The drawing under review shows one solid part. Ordinate dimensions are in mm from its lowest x, y, z. A direction names the side the tool comes from. Coordinates: 2 decimals unless noted, no trailing zeros. Write each loop counter-clockwise with the first axis right and the second up, starting at its lowest first coordinate (ties: lowest second). Pieces come first, ordered by that corner, then holes. Notation, with made-up numbers: (63.25, 43.5) -> (74.25, 43.5) arc R20 ccw to (74.25, 64.5) -> close; hole circle Ø9 at (-9.5, 22.25). An arc over 180 degrees is marked (long way). One line per question, with ' | ' between items. Start each with the question number.
Q1. Add section A-A on y = 95.5. State the section outline as (x, z) points (3 decimals).
Q2. Wall thickness on probe 1 along Y at (x, z) = (10.5, 54.5) (3 decimals); probe 2 along Z at (x, y) = (18, 133.5); probe 3 along Z at (x, y) = (13.25, 130.5): over which ranges is each line inside the solid? List them lowest first.
Q3. Draft analysis for pull direction Y (two halves, no side actions). For the marked faces 3, 4 and 5, state which applies: pulls with the +Y half, pulls with the -Y half, needs draft (parallel to the pull), parting line crosses it, or undercut.
Q4. Add section B-B on x = 9.25. State the section outline as (y, z) points (3 decimals), and give its area (3 significant figures).
Q5. For the marked faces 1 and 2, list the 3-axis set-ups (+Z, -Z, +X, -X, +Y, -Y) from which the entire face can be reached by the end or side of a thin tool; tool diameter is ignored.
Q6. For P1, Ø3.5, axis at x = 18, y = 137, coming from the +Z side; P2, Ø10.5, axis at y = 92, z = 28.5, coming from the +X side (3 decimals), all flat-tipped, find the tip position at first contact; note any pin that passes through.
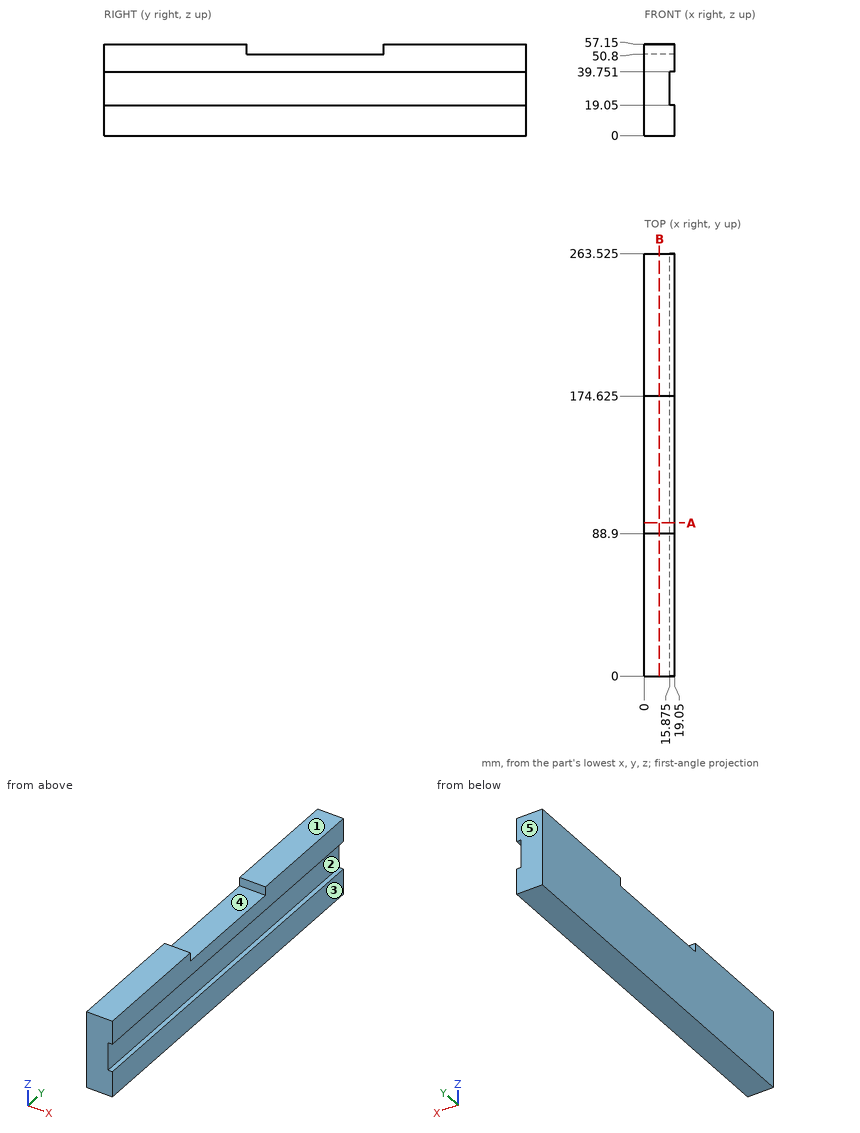
Output values:
1) outline: (0, 0) -> (19.05, 0) -> (19.05, 19.05) -> (15.875, 19.05) -> (15.875, 39.751) -> (19.05, 39.751) -> (19.05, 50.8) -> (0, 50.8) -> close
2) probe 1: y = 0 to 88.9, 174.625 to 263.525 | probe 2: z = 0 to 19.05, 39.75 to 50.8 | probe 3: z = 0 to 50.8
3) face 3: needs draft | face 4: undercut | face 5: pulls with the +Y half
4) outline: (0, 0) -> (263.525, 0) -> (263.525, 57.15) -> (174.625, 57.15) -> (174.625, 50.8) -> (88.9, 50.8) -> (88.9, 57.15) -> (0, 57.15) -> close | area: 14,500 mm2
5) face 1: +Z, +X, -X, +Y, -Y | face 2: +X, +Y, -Y
6) P1: stops at z = 50.8 | P2: stops at x = 15.875
